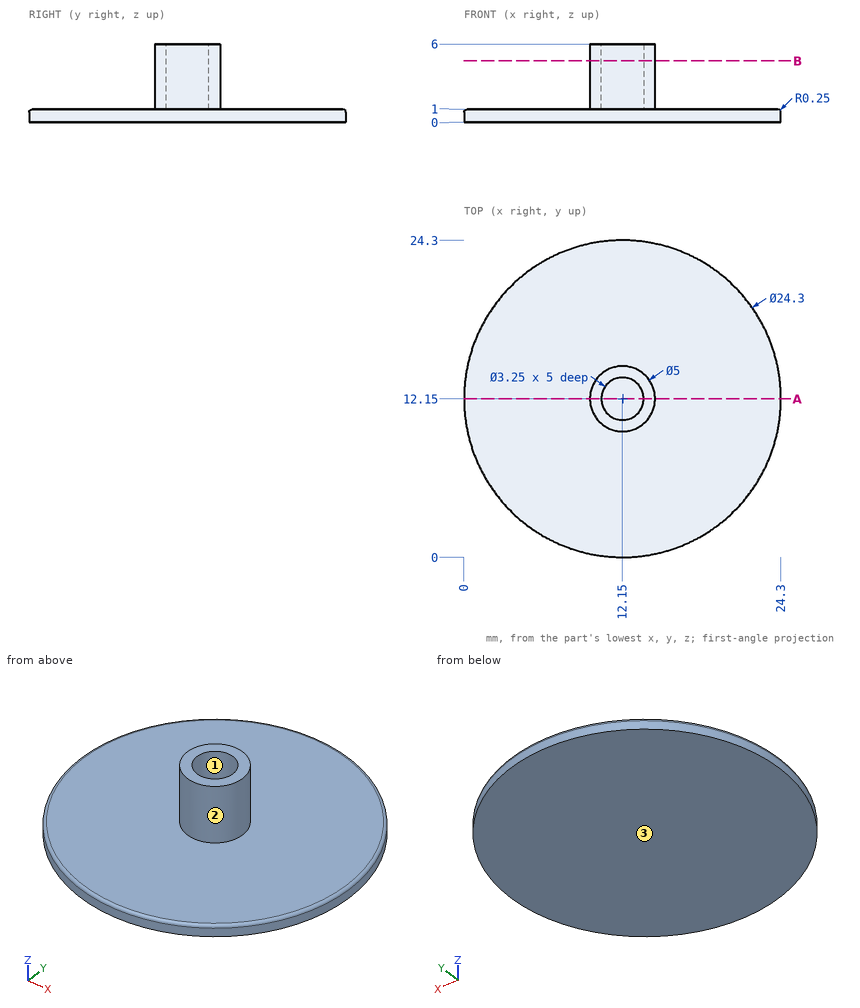
Answer from the drawing. Dimensions are ordinates in mm from the lowest x, y and z of the part. Round coordinates to 2 decimals unless told otherwise and drop trailing zeros. Loops run counter-clockwise (first coordinate to the right, second up) from the corner with the lowest first, then second, coordinate; pieces in that order, holes last.
1) A cutting plane is placed at B-B on z = 4.7. Determine the outline of the cut face in (x, y) (3 decimals), plus the area to 3 significant figures.
Outcome:
outline: circle Ø5 at (12.15, 12.15); hole circle Ø3.25 at (12.15, 12.15)
area: 11.3 mm2
2) Given P1, Ø1, axis at x = 15, y = 17.5, coming from the +Z side; P2, Ø2, axis at x = 12.5, z = 4, coming from the +Y side; P3, Ø3.5, axis at x = 11.5, y = 12.5, coming from the +Z side; P4, Ø1.5, axis at y = 2.5, z = 0.5, coming from the -X side, each flat-ended and moving along its own axis, determine where each tip first touches the part or whether it passes through.
Outcome:
P1: stops at z = 1
P2: stops at y = 14.65
P3: stops at z = 6
P4: stops at x = 3.88
3) Consider line 1 (Y direction, x = 12.15, z = 3.1) (3 decimals); line 2 (Z direction, x = 19.25, y = 14.5); line 3 (X direction, y = 14, z = 5.3). Determine where each line is inside the solid, lowest interval first.
Outcome:
line 1: y = 9.65 to 10.525, 13.775 to 14.65
line 2: z = 0 to 1
line 3: x = 10.47 to 13.83
4) A cutting plane is placed at A-A on y = 12.15. Determine the outline of the cut face in (x, z) (3 decimals), plus the area to 3 significant figures.
Outcome:
outline: (0, 0) - (24.3, 0) - (24.3, 0.75) arc R0.25 ccw to (24.05, 1) - (14.65, 1) - (14.65, 6) - (13.775, 6) - (13.775, 1) - (10.525, 1) - (10.525, 6) - (9.65, 6) - (9.65, 1) - (0.25, 1) arc R0.25 ccw to (0, 0.75) - close
area: 33.0 mm2
5) For a pull along X with two mould halves and no side action, classify the marked faces 1, 2 and 3 as released by +X, released by -X, zero draft, split by the parting line, or undercut.
Outcome:
face 1: undercut
face 2: split by the parting line
face 3: zero draft
